```python
from build123d import *

# Parameters (mm, degrees)
BOSS_EXTRUDE1_DEPTH = 0.515
SKETCH2_R           = 5.5
BOSS_EXTRUDE2_DEPTH = 0.01
SKETCH3_R           = 3.75
BOSS_EXTRUDE5_DEPTH = 0.525
BOSS_EXTRUDE6_DEPTH = 0.01
SKETCH6_R           = 0.5
CUT_EXTRUDE1_DEPTH  = 96.72347361
LPATTERN1_COUNT     = 15
LPATTERN1_PITCH     = 2.55
SKETCH7_R           = 2.275
SKETCH7_R_2         = 1.25
CUT_EXTRUDE2_DEPTH  = 96.72347361
SKETCH8_R           = 1.25
CUT_EXTRUDE3_DEPTH  = 96.72347361
SKETCH9_R           = 1.25
CUT_EXTRUDE4_DEPTH  = 96.72347361
SKETCH10_R          = 1.25
CUT_EXTRUDE5_DEPTH  = 96.72347361
SKETCH11_R          = 1.25
CUT_EXTRUDE6_DEPTH  = 96.72347361
SKETCH12_R          = 1.25
CUT_EXTRUDE7_DEPTH  = 96.72347361
SKETCH13_R          = 1.25
CUT_EXTRUDE8_DEPTH  = 96.72347361
SKETCH14_R          = 1.25
CUT_EXTRUDE9_DEPTH  = 96.72347361
SKETCH15_R          = 1.25
CUT_EXTRUDE10_DEPTH = 96.72347361
SKETCH16_R          = 1.25
CUT_EXTRUDE11_DEPTH = 96.72347361
SKETCH17_R          = 1.25
CUT_EXTRUDE12_DEPTH = 96.72347361


with BuildPart() as part:
    # Sketch1 → Boss-Extrude1 (new, symmetric)
    with BuildSketch(Plane.XY):
        with BuildLine():
            Line((0, 0), (55.75, 0))
            Line((55.75, 0), (58.15, 1.25))
            Line((58.15, 1.25), (81.25, 1.25))
            Line((81.25, 1.25), (81.25, -37.85))
            Line((81.25, -37.85), (65.45, -37.85))
            ThreePointArc((65.45, -37.85), (56.43438854, -41.58438854), (52.7, -50.6))
            Line((52.7, -50.6), (21.8, -50.6))
            Line((21.8, -50.6), (21.8, -41.4))
            Line((21.8, -41.4), (19.042567568, -38.75))
            Line((19.042567568, -38.75), (8.792567568, -38.75))
            Line((8.792567568, -38.75), (0, -30.3))
            Line((0, -30.3), (0, 0))
        make_face()
    extrude(amount=BOSS_EXTRUDE1_DEPTH, both=True)

    # Sketch2 → Boss-Extrude2 (add)
    with BuildSketch(Plane.XY.offset(0.515)):
        with Locations(Location((66.25, -4.5, 0), (0, 0, 180))):
            Circle(SKETCH2_R)
        with Locations(Location((73.15, -18.935719587, 0), (0, 0, 180))):
            Circle(SKETCH2_R)
        with Locations(Location((58.696235763, -25.844344587, 0), (0, 0, 180))):
            Circle(SKETCH2_R)
        with Locations(Location((51.796235763, -11.408625, 0), (0, 0, 180))):
            Circle(SKETCH2_R)
    extrude(amount=BOSS_EXTRUDE2_DEPTH)

    # Sketch3 → Boss-Extrude5 (add, through all)
    with BuildSketch(Plane.XY):
        with Locations((15, -14.375)):
            Circle(SKETCH3_R)
        with Locations((15, -32.625)):
            Circle(SKETCH3_R)
        with Locations((24.125, -23.5)):
            Circle(SKETCH3_R)
        with Locations((5.875, -23.5)):
            Circle(SKETCH3_R)
    extrude(amount=BOSS_EXTRUDE5_DEPTH)

    # Sketch5 → Boss-Extrude6 (add)
    with BuildSketch(Plane.XY.offset(0.515)):
        Polygon((32.918861679, -40.773499762), (23.3, -45.573499762), (25.309302326, -49.6), (34.928164005, -44.8), align=None)
        Polygon((38.3, -45.573499762), (40.309302326, -49.6), (49.928164005, -44.8), (47.918861679, -40.773499762), align=None)
    extrude(amount=BOSS_EXTRUDE6_DEPTH)

    # Sketch6 → Cut-Extrude1 (cut, through all)
    with BuildSketch(Plane.XY.offset(0.515)):
        with Locations((57.25, -1)):
            Circle(SKETCH6_R)
    cut_extrude1 = extrude(amount=-CUT_EXTRUDE1_DEPTH, mode=Mode.SUBTRACT)

    # LPattern1: Cut-Extrude1 ×15
    with Locations(*[(-i * LPATTERN1_PITCH, 0, 0) for i in range(1, LPATTERN1_COUNT)]):
        add(cut_extrude1, mode=Mode.SUBTRACT)

    # Sketch7 → Cut-Extrude2 (cut, through all)
    with BuildSketch(Plane.XY.offset(0.515)):
        with Locations((67.5, -34.1)):
            Circle(SKETCH7_R)
        with Locations((78.5, -31)):
            Circle(SKETCH7_R_2)
    extrude(amount=-CUT_EXTRUDE2_DEPTH, mode=Mode.SUBTRACT)

    # Sketch8 → Cut-Extrude3 (cut, through all)
    with BuildSketch(Plane.XY.offset(0.515)):
        with Locations((78.25, -8.25)):
            Circle(SKETCH8_R)
    extrude(amount=-CUT_EXTRUDE3_DEPTH, mode=Mode.SUBTRACT)

    # Sketch9 → Cut-Extrude4 (cut, through all)
    with BuildSketch(Plane.XY.offset(0.515)):
        with Locations((73.05, -7.75)):
            Circle(SKETCH9_R)
    extrude(amount=-CUT_EXTRUDE4_DEPTH, mode=Mode.SUBTRACT)

    # Sketch10 → Cut-Extrude5 (cut, through all)
    with BuildSketch(Plane.XY.offset(0.515)):
        with Locations((44.75, -7.5)):
            Circle(SKETCH10_R)
    extrude(amount=-CUT_EXTRUDE5_DEPTH, mode=Mode.SUBTRACT)

    # Sketch11 → Cut-Extrude6 (cut, through all)
    with BuildSketch(Plane.XY.offset(0.515)):
        with Locations((51.75, -22)):
            Circle(SKETCH11_R)
    extrude(amount=-CUT_EXTRUDE6_DEPTH, mode=Mode.SUBTRACT)

    # Sketch12 → Cut-Extrude7 (cut, through all)
    with BuildSketch(Plane.XY.offset(0.515)):
        with Locations((37.8, -41.6)):
            Circle(SKETCH12_R)
    extrude(amount=-CUT_EXTRUDE7_DEPTH, mode=Mode.SUBTRACT)

    # Sketch13 → Cut-Extrude8 (cut, through all)
    with BuildSketch(Plane.XY.offset(0.515)):
        with Locations((30.292567568, -36.6)):
            Circle(SKETCH13_R)
    extrude(amount=-CUT_EXTRUDE8_DEPTH, mode=Mode.SUBTRACT)

    # Sketch14 → Cut-Extrude9 (cut, through all)
    with BuildSketch(Plane.XY.offset(0.515)):
        with Locations((25.25, -34.1)):
            Circle(SKETCH14_R)
    extrude(amount=-CUT_EXTRUDE9_DEPTH, mode=Mode.SUBTRACT)

    # Sketch15 → Cut-Extrude10 (cut, through all)
    with BuildSketch(Plane.XY.offset(0.515)):
        with Locations((30.75, -14)):
            Circle(SKETCH15_R)
    extrude(amount=-CUT_EXTRUDE10_DEPTH, mode=Mode.SUBTRACT)

    # Sketch16 → Cut-Extrude11 (cut, through all)
    with BuildSketch(Plane.XY.offset(0.515)):
        with Locations((2.5, -7.5)):
            Circle(SKETCH16_R)
    extrude(amount=-CUT_EXTRUDE11_DEPTH, mode=Mode.SUBTRACT)

    # Sketch17 → Cut-Extrude12 (cut, through all)
    with BuildSketch(Plane.XY.offset(0.515)):
        with Locations((4, -13)):
            Circle(SKETCH17_R)
    extrude(amount=-CUT_EXTRUDE12_DEPTH, mode=Mode.SUBTRACT)


solid = part.part
```
Can you work these out from the model? Positions are in its coordinate system, mm. Coordinates: 2 decimals unless noted, no trailing zeros. Loops run counter-clockwise (first coordinate to the right, second up) from the corner with the lowest first, then second, coordinate; pieces in that order, holes last. Notation, with made-up numbers: (27.5, 62) -> (66.5, 62) arc R16 cw to (66.5, 79) -> close; hole circle Ø1 at (60, -30.5). An arc over 180 degrees is marked (long way). Answer as a JSON object with one key per item and string values.
1) For P1, Ø8, axis at x = 27, y = -33, coming from the +Z side (3 decimals), with a flat end and sliding along its axis, tell me the tip position at first contact or that it passes through.
Results:
{"P1": "stops at z = 0.515"}
2) Imagine slicing it at A-A (x = 15). Please give me the cut outline in (y, z) (3 decimals), then the cut area to 3 significant figures.
Results:
{"outline": "(-38.75, -0.515) -> (0, -0.515) -> (0, 0.515) -> (-10.625, 0.515) -> (-10.625, 0.525) -> (-18.125, 0.525) -> (-18.125, 0.515) -> (-28.875, 0.515) -> (-28.875, 0.525) -> (-36.375, 0.525) -> (-36.375, 0.515) -> (-38.75, 0.515) -> close", "area": "40.1 mm^2"}
3) If I drill on line 1 (Y direction, x = 31.75, z = 0.1); line 2 (Y direction, x = 9, z = -0.25); line 3 (Z direction, x = 17.5, y = -19.5) (3 decimals), over which ranges is the centre line in solid material (lowest first)?
Results:
{"line 1": "y = -50.6 to -14.75, -13.25 to -1.5, -0.5 to 0", "line 2": "y = -38.75 to 0", "line 3": "z = -0.515 to 0.515"}
4) Imagine slicing it at C-C (z = 0.05). Count the separate pieces of the cut face and the enclosed holes in it, then the cut area to 3 significant figures.
Results:
{"separate pieces": "1", "enclosed holes": "27", "area": "3,440 mm^2"}
5) Imagine slicing it at B-B (y = -22). Please give me the cut outline in (x, z) (3 decimals), then the cut area to 3 significant figures.
Results:
{"outline": "(0, -0.515) -> (50.5, -0.515) -> (50.5, 0.515) -> (27.562, 0.515) -> (27.562, 0.525) -> (20.688, 0.525) -> (20.688, 0.515) -> (9.312, 0.515) -> (9.312, 0.525) -> (2.438, 0.525) -> (2.438, 0.515) -> (0, 0.515) -> close; (53, -0.515) -> (81.25, -0.515) -> (81.25, 0.515) -> (77.717, 0.515) -> (77.717, 0.525) -> (68.583, 0.525) -> (68.583, 0.515) -> (62.63, 0.515) -> (62.63, 0.525) -> (54.763, 0.525) -> (54.763, 0.515) -> (53, 0.515) -> close", "area": "81.4 mm^2"}
6) Thinking about a two-plate mould opening in Y: for faces 1 (the face through (31.422, -12.946, 0.007)), 2 (the face through (44, -45, 0.525)), 3 (the face through (56.53, -41.49, 0.01)), 4 (the face through (25.09, -32.86, 0.01)), which applies, pulls with the +Y half, pulls with the -Y half, needs draft (parallel to the pull), parting line crosses it, or undercut?
Results:
{"face 1": "undercut", "face 2": "needs draft", "face 3": "pulls with the -Y half", "face 4": "undercut"}
